from build123d import *

# Parameters (mm, degrees)
F0_W     = 30
F0_H     = 30
F1_DEPTH = 2
F0_R     = 2
F3_DEPTH = 5
F4_DEPTH = 25
F2_R     = 1.5
F6_DEPTH = 15
F7_DEPTH = 15


# Not quite as in the source:
# - a feature names something its author has since deleted; it is built from what else it names


with BuildPart() as f1:
    # F0 (on Top) → F1 (new body)
    with BuildSketch(Plane.XY):
        with Locations((0, 6.2995284576)):
            Rectangle(F0_W, F0_H)
        with BuildLine():
            ThreePointArc((-10, 5), (-9.267766953, 6.767766953), (-7.5, 7.5))
            ThreePointArc((-7.5, 7.5), (-5.732233047, 6.767766953), (-5, 5))
            Line((-5, 5), (-5, 0))
            ThreePointArc((-5, 0), (-5.732233047, -1.767766953), (-7.5, -2.5))
            ThreePointArc((-7.5, -2.5), (-9.267766953, -1.767766953), (-10, 0))
            Line((-10, 0), (-10, 5))
        make_face(mode=Mode.SUBTRACT)
        with BuildLine():
            Line((5, 0), (5, 5))
            ThreePointArc((5, 5), (5.732233047, 6.767766953), (7.5, 7.5))
            ThreePointArc((7.5, 7.5), (9.267766953, 6.767766953), (10, 5))
            Line((10, 5), (10, 0))
            ThreePointArc((10, 0), (9.267766953, -1.767766953), (7.5, -2.5))
            ThreePointArc((7.5, -2.5), (5.732233047, -1.767766953), (5, 0))
        make_face(mode=Mode.SUBTRACT)
    extrude(amount=F1_DEPTH)

    # F0 (on Top) → F3 (join)
    with BuildSketch(Plane.XY):
        with BuildLine():
            ThreePointArc((7.5, 7.5), (5.732233047, 6.767766953), (5, 5))
            Line((5, 5), (5, 0))
            ThreePointArc((5, 0), (5.732233047, -1.767766953), (7.5, -2.5))
            ThreePointArc((7.5, -2.5), (9.267766953, -1.767766953), (10, 0))
            Line((10, 0), (10, 5))
            ThreePointArc((10, 5), (9.267766953, 6.767766953), (7.5, 7.5))
        make_face()
        with Locations((7.5, 0)):
            Circle(F0_R, mode=Mode.SUBTRACT)
        with BuildLine():
            ThreePointArc((-5, 5), (-5.732233047, 6.767766953), (-7.5, 7.5))
            ThreePointArc((-7.5, 7.5), (-9.267766953, 6.767766953), (-10, 5))
            Line((-10, 5), (-10, 0))
            ThreePointArc((-10, 0), (-9.267766953, -1.767766953), (-7.5, -2.5))
            ThreePointArc((-7.5, -2.5), (-5.732233047, -1.767766953), (-5, 0))
            Line((-5, 0), (-5, 5))
        make_face()
        with Locations((-7.5, 0)):
            Circle(F0_R, mode=Mode.SUBTRACT)
    extrude(amount=F3_DEPTH)

    # F0 (on Top) → F4 (join)
    with BuildSketch(Plane.XY):
        with Locations((7.5, 0)):
            Circle(F0_R)
        with Locations((-7.5, 0)):
            Circle(F0_R)
    extrude(amount=F4_DEPTH)

    # F2 (on Front) → F5 (revolve)
    with BuildSketch(Plane.XZ):
        with BuildLine():
            ThreePointArc((15, 50), (10.6066017178, 60.6066017178), (0, 65))
            Line((0, 65), (0, 46.9528951543))
            ThreePointArc((0, 46.9528951543), (3.0017193367, 48.1526751529), (4.2698885231, 51.1261475231))
            ThreePointArc((4.2698885231, 51.1261475231), (4.3593428406, 46.0758998678), (0, 43.5245995224))
            Line((0, 43.5245995224), (0, 15))
            ThreePointArc((0, 15), (10.6066017178, 19.3933982822), (15, 30))
            Line((15, 30), (15, 50))
        make_face()
        with Locations((6, 57.3495886624)):
            Circle(F2_R, mode=Mode.SUBTRACT)
        with Locations((6, 57.3495886624)):
            Circle(F2_R)
        with BuildLine():
            ThreePointArc((4.2698885231, 51.1261475231), (3.0017193367, 48.1526751529), (0, 46.9528951543))
            Line((0, 46.9528951543), (0, 43.5245995224))
            ThreePointArc((0, 43.5245995224), (4.3593428406, 46.0758998678), (4.2698885231, 51.1261475231))
        make_face()
    revolve(axis=Axis((0, 0, 40), (0, 0, -1)))

    # F2 (on Front) → F6 (cut, symmetric)
    with BuildSketch(Plane.XZ):
        with Locations((6, 57.3495886624)):
            Circle(F2_R)
        with Locations((-6, 57.3495886624)):
            Circle(F2_R)
    extrude(amount=F6_DEPTH, both=True, mode=Mode.SUBTRACT)

    # F2 (on Front) → F7 (cut, symmetric)
    with BuildSketch(Plane.XZ):
        with BuildLine():
            ThreePointArc((4.2698885231, 51.1261475231), (3.0017193367, 48.1526751529), (0, 46.9528951543))
            Line((0, 46.9528951543), (0, 43.5245995224))
            ThreePointArc((0, 43.5245995224), (4.3593428406, 46.0758998678), (4.2698885231, 51.1261475231))
        make_face()
        with BuildLine():
            Line((0, 43.5245995224), (0, 46.9528951543))
            ThreePointArc((0, 46.9528951543), (-2.9917232596, 48.2573678623), (-4.1542744288, 51.3070452037))
            ThreePointArc((-4.1542744288, 51.3070452037), (-4.4109085463, 46.1700537495), (0, 43.5245995224))
        make_face()
    extrude(amount=F7_DEPTH, both=True, mode=Mode.SUBTRACT)


solid = f1.part
Can you work these out from the model? Positions are in its coordinate system, mm. A direction names the side the tool comes from. Round coordinates to 2 decimals unless told otherwise and drop trailing zeros. Write each loop counter-clockwise with the first axis right and the second up, starting at its lowest first coordinate (ties: lowest second). Pieces come first, ordered by that corner, then holes. Notation, with made-up numbers: (10, -11) - (14, -11) arc R23 ccw to (14, 28) - close; hole circle Ø1 at (52, 33). An arc over 180 degrees is marked (long way). Write each question's results on one line, items separated by ' | '. Start each with the question number.
1) Suppose I cut it at B-B (y = 16.5). List the corners of the cut face in (x, z) for me.
2) Suppose I cut it at C-C (z = 32). List the corners of the cut face in (x, y) for me.
3) Suppose I cut it at D-D (z = 45.5). List the corners of the cut face in (x, y) for me.
4) Which directions (+Z, -Z, +X, -X, +Y, -Y) give clear straight access to the entire face, cutting with the end or side of a thin tool? Please do faces 1 (the cylindrical face through (0, 15, 49)), 2 (the cylindrical face through (-9.498, 0.088, 11.602)), 3 (the flat face through (0, -8.7, 1)).
5) Please list where these lines run through material, in increasing order: line 1 (X direction, y = 7, z = 58); line 2 (X direction, y = 6, z = 58); line 3 (Z direction, x = -6, y = -3).
6) Suppose I cut it at A-A (z = 13). List the corners of the cut face in (x, y) for me.
7) For pin 1 Ø10 at (x, y) = (-4, 11.5) entering from -Z; pin 2 Ø3.5 at (y, z) = (3.5, 4) entering from +X; pin 3 Ø0.6 at (x, z) = (-5.5, 1.5) entering from -Y; pin 4 Ø1 at (x, y) = (-11, 16.5) entering from +Z, each with a flat end and sliding along its axis, tell me the tip position at first contact or that it passes through.
8) We'd pull the mould along X, two halves only. Please class faces 4 (the flat face through (0, 7, 0)), 5 (the cylindrical face through (0.06, -0.21, 46.953)), 6 (the flat face through (-15, 6, 1)): released by +X, released by -X, zero draft, split by the parting line, or undercut.
Here are the results:
1) outline: (-15, 0) - (15, 0) - (15, 2) - (-15, 2) - close
2) outline: circle Ø30 at (0, 0)
3) outline: (-3.98, -14.46) - (-3.98, 14.46) arc R15 ccw to start; (3.98, -14.46) arc R15 ccw to (3.98, 14.46) - close
4) face 1: +Z, +Y | face 2: none | face 3: -Z, +X, -X, -Y
5) line 1: x = -10.58 to -7.35, -4.65 to 4.65, 7.35 to 10.58 | line 2: x = -11.18 to -7.35, -4.65 to 4.65, 7.35 to 11.18 | line 3: z = 0 to 2, 16.58 to 55.85, 58.85 to 63.42
6) outline: circle Ø4 at (-7.5, 0); circle Ø4 at (7.5, 0)
7) pin 1: stops at z = 0 | pin 2: stops at x = 10 | pin 3: stops at y = -8.7 | pin 4: stops at z = 2
8) face 4: zero draft | face 5: undercut | face 6: released by -X
